For this review, take the finished solid that the model builds, in its own axes (mm). A direction names the side the tool comes from. Round coordinates to 2 decimals unless told otherwise and drop trailing zeros. Loops run counter-clockwise (first coordinate to the right, second up) from the corner with the lowest first, then second, coordinate; pieces in that order, holes last.
1. To check wall thickness, follow line 1 along Y through (x, z) = (342.43, -1.05); line 2 along Z through (x, y) = (325, 9); line 3 along Y through (x, z) = (364.93, -1) (3 decimals). State the ranges of each line that lie inside material, in increasing order.
2. Draft analysis for pull direction X (two halves, no side actions). For faces 1 (the flat face through (174, 16, -8)), 2 (the cylindrical face through (-12.85, -1.97, -1.48)), 3 (the flat face through (291.222, -1.784, -1.521)), state which applies: released by +X, released by -X, zero draft, split by the parting line, or undercut.
3. Consider section C-C on x = 306.5. State the section outline as (y, z) points, then the cut area to 3 significant figures.
4. Consider section A-A on x = 33.5. State the section outline as (y, z) points.
5. Consider section B-B on z = -8.25. State the section outline as (x, y) points, then the cut area to 3 significant figures.
6. Tool access review of faces 4 (the flat face through (174, 13, -8)), 5 (the flat face through (170.38, -2.43, -1.52)), 6 (the flat face through (181, -7, 0)): name each direction out of +Z, -Z, +X, -X, +Y, -Y from which nothing blocks a thin tool from reaching the whole face with its end or side.
7. Clearance check with flat-ended pins moving along their axes: pin 1 Ø12 at (x, y) = (123.5, -2) entering from -Z; pin 2 Ø1.5 at (x, z) = (56, -1.5) entering from +Y; pin 3 Ø6 at (y, z) = (-11, -5) entering from -X. State where each tip first meets the part, or that it passes through.
from build123d import *

# Parameters (mm, degrees)
BASE_FLANGE1_DEPTH            = 3
EDGE_FLANGE2_STRIP_W          = 13.4732
EDGE_FLANGE2_STRIP_H          = 3
EDGE_FLANGE2_STRIP_CUT_DEPTH  = 349.93
EDGE_FLANGE2_RELIEF_W         = 14.9732
EDGE_FLANGE2_RELIEF_H         = 1.5
EDGE_FLANGE2_RELIEF_CUT_DEPTH = 3
EDGE_FLANGE2_DEPTH            = 349.93
CUT_EXTRUDE1_DEPTH            = 372.108077115
CUT_EXTRUDE1_DEPTH_BACK       = 372.108077115
SKETCH22_R                    = 4.075
SKETCH22_R_2                  = 11.075
SKETCH22_R_3                  = 1.575
CUT_EXTRUDE2_DEPTH            = 372.108077115
CUT_EXTRUDE2_DEPTH_BACK       = 372.108077115
FILLET1_R                     = 2
CUT_EXTRUDE3_DEPTH            = 372.108077115
CUT_EXTRUDE3_DEPTH_BACK       = 372.108077115
SKETCH24_W                    = 100
SKETCH24_H                    = 5.2366
FILLET2_R                     = 1.5


# Sheet-metal steps are written as plain solids
with BuildPart() as part:
    # Sketch1 → Base-Flange1 (new body)
    with BuildSketch(Plane.XY):
        with BuildLine():
            Line((0, 13), (349.93, 13))
            ThreePointArc((349.93, 13), (366.008670386, -18.89438349), (330.805412842, -12.852364139))
            Line((330.805412842, -12.852364139), (0, -13))
            ThreePointArc((0, -13), (-13, 0), (0, 13))
        make_face()
    extrude(amount=-BASE_FLANGE1_DEPTH)

    # Edge-Flange2 strip (across the edge) → Edge-Flange2 strip cut (cut)
    with BuildSketch(Plane(origin=(0, 13, -3), x_dir=(0, -1, 0), z_dir=(1, 0, 0))):
        with Locations((-6, -1.5)):
            Rectangle(EDGE_FLANGE2_STRIP_W, EDGE_FLANGE2_STRIP_H)
    extrude(amount=EDGE_FLANGE2_STRIP_CUT_DEPTH, mode=Mode.SUBTRACT)

    # Edge-Flange2 relief (on the sheet) → Edge-Flange2 relief cut (cut)
    with BuildSketch(Plane(origin=(0, 12.2634, -3), x_dir=(0, -1, 0), z_dir=(0, 0, -1))):
        with Locations((-5.9866, 0.75)):
            Rectangle(EDGE_FLANGE2_RELIEF_W, EDGE_FLANGE2_RELIEF_H)
        with Locations((-5.9866, -350.68)):
            Rectangle(EDGE_FLANGE2_RELIEF_W, EDGE_FLANGE2_RELIEF_H)
    extrude(amount=-EDGE_FLANGE2_RELIEF_CUT_DEPTH, mode=Mode.SUBTRACT)

    # Edge-Flange2 section (across the edge) → Edge-Flange2 (add)
    with BuildSketch(Plane(origin=(0, 13, -3), x_dir=(0, -1, 0), z_dir=(1, 0, 0))):
        with BuildLine():
            Line((-3, 0.7366), (-3, 9))
            Line((-3, 9), (0, 9))
            Line((0, 9), (0, 0.7366))
            ThreePointArc((0, 0.7366), (0.215745145, 0.215745145), (0.7366, 0))
            Line((0.7366, 0), (0.7366, -3))
            ThreePointArc((0.7366, -3), (-1.905575199, -1.905575199), (-3, 0.7366))
        make_face()
    extrude(amount=EDGE_FLANGE2_DEPTH)

    # Sketch22 → Cut-Extrude1 (cut, two sides: drawn at the far end of the back side and taken through both)
    with BuildSketch(Plane.XY.offset(-CUT_EXTRUDE1_DEPTH_BACK)):
        Circle(SKETCH22_R)
        with Locations((349.93, -7)):
            Circle(SKETCH22_R_2)
        with Locations((364.93, -7)):
            Circle(SKETCH22_R_3)
        with Locations((342.43, 5.990381057)):
            Circle(SKETCH22_R_3)
        with Locations((342.43, -19.990381057)):
            Circle(SKETCH22_R_3)
    extrude(amount=CUT_EXTRUDE1_DEPTH + CUT_EXTRUDE1_DEPTH_BACK, mode=Mode.SUBTRACT)

    # Sketch23 → Cut-Extrude2 (cut, two sides: drawn at the far end of the back side and taken through both)
    with BuildSketch(Plane.XY.offset(-CUT_EXTRUDE2_DEPTH_BACK)):
        Polygon((12.5, 6.5), (12.5, -6.5), (111.651399385, -6.5), align=None)
        Polygon((327.5, 6.5), (227.5, 6.5), (327.5, -6.5), align=None)
        Polygon((50.961538462, 6.5), (163.478075869, -8.252338296), (180.961538462, 6.5), align=None)
        Polygon((173.308112114, -6.5), (288.714823182, -6.5), (188.714823182, 6.5), align=None)
    extrude(amount=CUT_EXTRUDE2_DEPTH + CUT_EXTRUDE2_DEPTH_BACK, mode=Mode.SUBTRACT)

    # Fillet1
    fillet1_edges = [part.edges().sort_by_distance(p)[0] for p in [
        (12.5, 6.5, -1.5),
        (288.714823182, -6.5, -1.5),
        (173.308112114, -6.5, -1.5),
        (188.714823182, 6.5, -1.5),
        (163.478075869, -8.252338296, -1.5),
        (50.961538462, 6.5, -1.5),
        (180.961538462, 6.5, -1.5),
        (227.5, 6.5, -1.5),
        (0, 14.5, -12),
        (349.93, 14.5, -12),
        (327.5, -6.5, -1.5),
        (327.5, 6.5, -1.5),
        (111.651399385, -6.5, -1.5),
        (12.5, -6.5, -1.5),
    ]]
    fillet(fillet1_edges, radius=FILLET1_R)

    # Sketch24 → Cut-Extrude3 (cut, two sides: drawn at the far end of the back side and taken through both)
    with BuildSketch(Plane.XY.offset(-CUT_EXTRUDE3_DEPTH_BACK)):
        with Locations((50, 13.3817)):
            Rectangle(SKETCH24_W, SKETCH24_H)
        with Locations((299.93, 13.3817)):
            Rectangle(SKETCH24_W, SKETCH24_H)
    extrude(amount=CUT_EXTRUDE3_DEPTH + CUT_EXTRUDE3_DEPTH_BACK, mode=Mode.SUBTRACT)

    # Fillet2
    fillet2_edges = [part.edges().sort_by_distance(p)[0] for p in [
        (351.43, 12.943670675, -1.5),
        (-1.5, 12.91317157, -1.5),
        (100, 14.5, -12),
        (249.93, 14.5, -12),
    ]]
    fillet(fillet2_edges, radius=FILLET2_R)


solid = part.part
Resolved:
1. line 1: y = -25.54 to -21.57, -18.42 to -15.15, 1.15 to 4.42, 7.57 to 10.76
1. line 2: z = -3 to 0
1. line 3: y = -20.229 to -8.575, -5.425 to 6.229
2. face 1: zero draft
2. face 2: released by -X
2. face 3: undercut
3. outline: (-12.86, -3) - (-3.77, -3) - (-3.77, 0) - (-12.86, 0) - close; (6.5, -3) - (10.76, -3) - (10.76, 0) - (6.5, 0) - close
3. area: 40.1 mm2
4. outline: (-12.99, -3) - (-6.5, -3) - (-6.5, 0) - (-12.99, 0) - close; (3.75, -3) - (10.76, -3) - (10.76, 0) - (3.75, 0) - close
5. outline: (100, 13) - (249.93, 13) - (249.93, 16) - (100, 16) - close
5. area: 450 mm2
6. face 4: -Z, +X, -X, -Y
6. face 5: +Z, -Z
6. face 6: +Z, +X, -X, +Y, -Y
7. pin 1: stops at z = -3
7. pin 2: stops at y = 10.76
7. pin 3: stops at x = -9.6
